```python
from build123d import *

# Parameters (mm, degrees)
SKETCH_1_R      = 20
SKETCH_1_R_2    = 2.5
EXTRUDE_1_DEPTH = 6
SKETCH_2_R      = 9
EXTRUDE_2_DEPTH = 26
CHAMFER_1_SIZE  = 0.8
CHAMFER_2_SIZE  = 2


with BuildPart() as part:
    # 草图1 → 凸台-拉伸1 (new body)
    with BuildSketch(Plane(origin=(0, 0, 0), x_dir=(1, 0, 0), z_dir=(0, 1, 0))):
        with Locations(Location((0, 0, 0), (0, 0, 270))):
            Circle(SKETCH_1_R)
        with Locations(Location((-11.136931804, 11.136931804, 0), (0, 0, 270))):
            Circle(SKETCH_1_R_2, mode=Mode.SUBTRACT)
        with Locations(Location((11.136931804, 11.136931804, 0), (0, 0, 270))):
            Circle(SKETCH_1_R_2, mode=Mode.SUBTRACT)
        with Locations(Location((11.136931804, -11.136931804, 0), (0, 0, 270))):
            Circle(SKETCH_1_R_2, mode=Mode.SUBTRACT)
        with Locations(Location((-11.136931804, -11.136931804, 0), (0, 0, 270))):
            Circle(SKETCH_1_R_2, mode=Mode.SUBTRACT)
    extrude(amount=EXTRUDE_1_DEPTH)

    # 草图2 → 凸台-拉伸2 (add)
    with BuildSketch(Plane(origin=(0, 6, 0), x_dir=(1, 0, 0), z_dir=(0, 1, 0))):
        with Locations(Location((0, 0, 0), (0, 0, 90))):
            Circle(SKETCH_2_R)
        with BuildLine():
            Line((1.936491673, 3.5), (-1.936491673, 3.5))
            ThreePointArc((-1.936491673, 3.5), (-2.828427125, 2.828427125), (-3.5, 1.936491673))
            Line((-3.5, 1.936491673), (-3.5, -1.936491673))
            ThreePointArc((-3.5, -1.936491673), (-2.828427125, -2.828427125), (-1.936491673, -3.5))
            Line((-1.936491673, -3.5), (1.936491673, -3.5))
            ThreePointArc((1.936491673, -3.5), (2.828427125, -2.828427125), (3.5, -1.936491673))
            Line((3.5, -1.936491673), (3.5, 1.936491673))
            ThreePointArc((3.5, 1.936491673), (2.828427125, 2.828427125), (1.936491673, 3.5))
        make_face(mode=Mode.SUBTRACT)
    extrude(amount=EXTRUDE_2_DEPTH)

    # 倒角1
    chamfer_1_edges = [part.edges().sort_by_distance(p)[0] for p in [
        (0, 6, -20),
    ]]
    chamfer(chamfer_1_edges, length=CHAMFER_1_SIZE)

    # 倒角2
    chamfer_2_edges = [part.edges().sort_by_distance(p)[0] for p in [
        (0, 32, 9),
    ]]
    chamfer(chamfer_2_edges, length=CHAMFER_2_SIZE)


solid = part.part
```
For this review, take the finished solid that the model builds, in its own axes (mm). A direction names the side the tool comes from. Coordinates: 2 decimals unless noted, no trailing zeros. Write each loop counter-clockwise with the first axis right and the second up, starting at its lowest first coordinate (ties: lowest second). Pieces come first, ordered by that corner, then holes. Notation, with made-up numbers: (-37.5, 29.25) - (15.5, 29.25) arc R13 ccw to (15.5, 40.25) - close; hole circle Ø11 at (61, -25). An arc over 180 degrees is marked (long way). Put each result on its own line as item: value.
1. Add section A-A, the plane y = 26.5. Give the boundary of the cut face in (x, z), then the cut area to 3 significant figures.
Values found:
outline: circle Ø18 at (0, 0); hole (-3.5, -1.94) arc R4 ccw to (-1.94, -3.5) - (1.94, -3.5) arc R4 ccw to (3.5, -1.94) - (3.5, 1.94) arc R4 ccw to (1.94, 3.5) - (-1.94, 3.5) arc R4 ccw to (-3.5, 1.94) - close
area: 209 mm²
2. Add section D-D, the plane x = 10.5. Count the separate pieces of the cut face and the enclosed holes in it, then the cut area to 3 significant figures.
Values found:
separate pieces: 3
enclosed holes: 0
area: 145 mm²
3. Add section B-B, the plane x = 0. Give the boundary of the cut face in (y, z).
Values found:
outline: (0, -20) - (5.2, -20) - (6, -19.2) - (6, -9) - (30, -9) - (32, -7) - (32, -3.5) - (6, -3.5) - (6, 3.5) - (32, 3.5) - (32, 7) - (30, 9) - (6, 9) - (6, 19.2) - (5.2, 20) - (0, 20) - close
4. For pin 1 (6 mm diameter, centred on x = 11.5, z = -3, fed in from -Y); pin 2 (5.5 mm diameter, centred on x = 0, z = -0.5, fed in from +Y); pin 3 (6 mm diameter, centred on y = 17.5, z = -9.5, fed in from -X); pin 4 (8 mm diameter, centred on y = 17, z = -5, fed in from -X), all flat-tipped, find the tip position at first contact; note any pin that passes through.
Values found:
pin 1: y = 0
pin 2: y = 6
pin 3: x = -6.22
pin 4: x = -8.94
5. Mouldability with a two-part tool opening along Z and no side actions: class faces 3 (the cylindrical face through (-19.524, 2.564, -4.336)), 4 (the flat face through (-4, 6, 8.3)), 5 (the cylindrical face through (-2.839, 18.818, 2.817)) as released by +Z, released by -Z, zero draft, split by the parting line, or undercut.
Values found:
face 3: split by the parting line
face 4: zero draft
face 5: undercut
6. Machinability: for faces 1 (the flat face through (3, 32, -3)), 2 (the flat face through (0, 6, 0)), which of the approach directions +Z, -Z, +X, -X, +Y, -Y give a long, thin tool a straight path to every point of the face, cutting with its end or side? Answer none if there is none.
Values found:
face 1: +Z, -Z, +X, -X, +Y
face 2: +Y
7. Wall thickness on probe 1 along X at (y, z) = (26, 0); probe 2 along Y at (x, z) = (-4.5, -8); probe 3 along X at (y, z) = (25.5, -3): over which ranges is each line inside the solid? List them lowest first.
Values found:
probe 1: -9 to -3.5, 3.5 to 9
probe 2: 0 to 6
probe 3: -8.49 to -2.65, 2.65 to 8.49
8. Add section C-C, the plane z = 0. Give the boundary of the cut face in (x, y), then the cut area to 3 significant figures.
Values found:
outline: (-20, 0) - (20, 0) - (20, 5.2) - (19.2, 6) - (9, 6) - (9, 30) - (7, 32) - (3.5, 32) - (3.5, 6) - (-3.5, 6) - (-3.5, 32) - (-7, 32) - (-9, 30) - (-9, 6) - (-19.2, 6) - (-20, 5.2) - close
area: 521 mm²
